Can you work these out from the model? Positions are in its coordinate system, mm. A direction names the side the tool comes from. Coordinates: 2 decimals unless noted, no trailing zeros. Write each loop counter-clockwise with the first axis right and the second up, starting at its lowest first coordinate (ties: lowest second). Pieces come first, ordered by that corner, then holes.
```python
from build123d import *

# Parameters (mm, degrees)
SKETCH006_R            = 2.5
SKETCH006_R_2          = 38.75
PAD004_DEPTH           = 1.5
SKETCH007_W            = 1.5
SKETCH007_H            = 80
PAD005_DEPTH           = 1.5
LINEARPATTERN002_COUNT = 5
LINEARPATTERN002_PITCH = 15
SKETCH008_W            = 80
SKETCH008_H            = 1.5
PAD006_DEPTH           = 1.5
LINEARPATTERN003_COUNT = 5
LINEARPATTERN003_PITCH = 15
PAD007_DEPTH           = 3


with BuildPart() as part:
    # Sketch006 → Pad004 (new body)
    with BuildSketch(Plane.XY):
        with BuildLine():
            Line((40, -36), (40, 36))
            ThreePointArc((40, 36), (38.828427, 38.828427), (36, 40))
            Line((36, 40), (-36, 40))
            ThreePointArc((-36, 40), (-38.828427, 38.828427), (-40, 36))
            Line((-40, 36), (-40, -36))
            ThreePointArc((-40, -36), (-38.828427, -38.828427), (-36, -40))
            Line((-36, -40), (36, -40))
            ThreePointArc((36, -40), (38.828427, -38.828427), (40, -36))
        make_face()
        with Locations((-35.75, 35.75)):
            Circle(SKETCH006_R, mode=Mode.SUBTRACT)
        with Locations((35.75, 35.75)):
            Circle(SKETCH006_R, mode=Mode.SUBTRACT)
        with Locations((35.75, -35.75)):
            Circle(SKETCH006_R, mode=Mode.SUBTRACT)
        with Locations((-35.75, -35.75)):
            Circle(SKETCH006_R, mode=Mode.SUBTRACT)
        Circle(SKETCH006_R_2, mode=Mode.SUBTRACT)
    extrude(amount=PAD004_DEPTH)

    # Sketch007 → Pad005 (join)
    with BuildSketch(Plane.XY):
        with Locations((-30, 0)):
            Rectangle(SKETCH007_W, SKETCH007_H)
    pad005 = extrude(amount=PAD005_DEPTH)

    # LinearPattern002: Pad005 ×5
    with Locations(*[(i * LINEARPATTERN002_PITCH, 0, 0) for i in range(1, LINEARPATTERN002_COUNT)]):
        add(pad005)

    # Sketch008 → Pad006 (join)
    with BuildSketch(Plane.XY):
        with Locations((0, -30)):
            Rectangle(SKETCH008_W, SKETCH008_H)
    pad006 = extrude(amount=PAD006_DEPTH)

    # LinearPattern003: Pad006 ×5
    with Locations(*[(0, i * LINEARPATTERN003_PITCH, 0) for i in range(1, LINEARPATTERN003_COUNT)]):
        add(pad006)

    # Sketch009 (on Face137 of LinearPattern003) → Pad007 (join)
    with BuildSketch(Plane.XY.offset(1.5)):
        with BuildLine():
            Line((-40, 36), (-40, -36))
            ThreePointArc((-40, -36), (-38.828427, -38.828427), (-36, -40))
            Line((-36, -40), (36, -40))
            ThreePointArc((36, -40), (38.828427, -38.828427), (40, -36))
            Line((40, -36), (40, 36))
            ThreePointArc((40, 36), (38.828427, 38.828427), (36, 40))
            Line((36, 40), (-36, 40))
            ThreePointArc((-36, 40), (-38.828427, 38.828427), (-40, 36))
        make_face()
        with BuildLine():
            Line((-39, 36), (-39, -36))
            ThreePointArc((-39, -36), (-38.12132, -38.12132), (-36, -39))
            Line((-36, -39), (36, -39))
            ThreePointArc((36, -39), (38.12132, -38.12132), (39, -36))
            Line((39, -36), (39, 36))
            ThreePointArc((39, 36), (38.12132, 38.12132), (36, 39))
            Line((36, 39), (-36, 39))
            ThreePointArc((-36, 39), (-38.12132, 38.12132), (-39, 36))
        make_face(mode=Mode.SUBTRACT)
    extrude(amount=PAD007_DEPTH)


solid = part.part
```
1. If we section it at A-A, the plane z = 2.8: List the corners of the cut face in (x, y) for me.
2. If I drill on L1, parallel to Y at x = 35.75, z = 0.9; L2, parallel to Y at x = -30, z = 4.2, over which ranges is the centre line in solid material (lowest first)?
3. We'd pull the mould along X, two halves only. Please class faces 3 (the face through (-38.797, 38.859, 2.218)), 4 (the face through (37.974, -7.716, 0.74)), 5 (the face through (1, 40, 2)): released by +X, released by -X, zero draft, split by the parting line, or undercut.
4. If we section it at C-C, the plane y = -9: Count the separate pieces of the cut face and the enclosed holes in it, plus the area to 3 significant figures.
5. If we section it at D-D, the plane y = 32: List the corners of the cut face in (x, z) for me.
6. If we section it at B-B, the plane y = -28: List the corners of the cut face in (x, z) for me.
7. I'm going to push flat-ended pins straight in: P1, Ø10, axis at x = 6.5, y = 29.5, coming from the -Z side; P2, Ø1.5, axis at x = 12.5, y = -9, coming from the +Z side; P3, Ø6, axis at x = 24, y = -12.5, coming from the +Z side. Where does each tip first touch, or does it pass through?
8. Which directions (+Z, -Z, +X, -X, +Y, -Y) give clear straight access to the entire face, cutting with the end or side of a thin tool? Please do faces 1 (the face through (38.14, 38.1, 2.98)), 2 (the face through (-38.01, -7.53, 0.74)).
Answers:
1. outline: (-40, -36) arc R4 ccw to (-36, -40) - (36, -40) arc R4 ccw to (40, -36) - (40, 36) arc R4 ccw to (36, 40) - (-36, 40) arc R4 ccw to (-40, 36) - close; hole (-39, -36) arc R3 ccw to (-36, -39) - (36, -39) arc R3 ccw to (39, -36) - (39, 36) arc R3 ccw to (36, 39) - (-36, 39) arc R3 ccw to (-39, 36) - close
2. L1: y = -40 to -38.25, -33.25 to -14.25, -0.75 to 0.75, 14.25 to 33.25, 38.25 to 40
2. L2: y = -40 to -39, 39 to 40
3. face 3: released by -X
3. face 4: undercut
3. face 5: zero draft
4. separate pieces: 7
4. enclosed holes: 0
4. area: 24.2 mm2
5. outline: (-40, 0) - (-21.85, 0) - (-21.85, 1.5) - (-39, 1.5) - (-39, 4.5) - (-40, 4.5) - close; (-15.75, 0) - (-14.25, 0) - (-14.25, 1.5) - (-15.75, 1.5) - close; (-0.75, 0) - (0.75, 0) - (0.75, 1.5) - (-0.75, 1.5) - close; (14.25, 0) - (15.75, 0) - (15.75, 1.5) - (14.25, 1.5) - close; (21.85, 0) - (40, 0) - (40, 4.5) - (39, 4.5) - (39, 1.5) - (21.85, 1.5) - close
6. outline: (-40, 0) - (-26.79, 0) - (-26.79, 1.5) - (-39, 1.5) - (-39, 4.5) - (-40, 4.5) - close; (-15.75, 0) - (-14.25, 0) - (-14.25, 1.5) - (-15.75, 1.5) - close; (-0.75, 0) - (0.75, 0) - (0.75, 1.5) - (-0.75, 1.5) - close; (14.25, 0) - (15.75, 0) - (15.75, 1.5) - (14.25, 1.5) - close; (26.79, 0) - (40, 0) - (40, 4.5) - (39, 4.5) - (39, 1.5) - (26.79, 1.5) - close
7. P1: stops at z = 0
7. P2: passes through
7. P3: stops at z = 1.5
8. face 1: +Z
8. face 2: +Z, -Z
